Read the model definition and answer for the solid it produces. Units are mm, in the model's axes. Face numbers are marked on the shaded views. A direction names the side the tool comes from. Coordinates: 2 decimals unless noted, no trailing zeros. Write each loop counter-clockwise with the first axis right and the second up, starting at its lowest first coordinate (ties: lowest second). Pieces come first, ordered by that corner, then holes.
(1) The part is cut by section C-C, the plane z = 2.15. Determine the outline of the cut face in (x, y), and give its area (3 significant figures).
(2) The part is cut by section A-A, the plane x = 0.75. Determine the outline of the cut face in (y, z), and give its area (3 significant figures).
(3) Which of the six approach directions +Z, -Z, +X, -X, +Y, -Y give full straight-line access (tool end or side, diameter ignored) to the marked faces 4, 5 and 6?
(4) Straight lines are drawn through the part: line 1 along X through (y, z) = (5.25, 2.4); line 2 along Z through (x, y) = (-6, -1). For each, find the intervals that lie inside material, in ascending order.
(5) Given pin 1 (0.5 mm diameter, centred on x = 1.5, z = 2.5, fed in from +Y); pin 2 (4 mm diameter, centred on x = -1, y = -2, fed in from +Z), each flat-ended and moving along its own axis, determine where each tip first touches the part or whether it passes through.
(6) Determine the mould class of the marked faces 1, 2 and 3 for opening direction X: pulls with the +X half, pulls with the -X half, needs draft (parallel to the pull), parting line crosses it, or undercut.
(7) The part is cut by section B-B, the plane y = -3. Determine the outline of the cut face in (x, z).
Autodesk Fusion 360 part; units mm, degrees
sketch "Sketch1" plane through (0, 0, 0) normal (0, 0, 1) x (1, 0, 0)
  line L0 (-7.9, 7.9) -> (7.9, 7.9)
  line L1 (7.9, 7.9) -> (7.9, -7.9)
  line L2 (7.9, -7.9) -> (-7.9, -7.9)
  line L3 (-7.9, -7.9) -> (-7.9, 7.9)
  line L4 (-7.9, 7.9) -> (7.9, -7.9) construction
  line L5 (7.9, 7.9) -> (-7.9, -7.9) construction
  dimension "d1" = 15.8
extrude "Extrude1" add sketch "Sketch1" along normal blind 3.3
shell "Shell1" thickness 1.55 removed faces 1 at (-2.6333, 2.6333, 3.3)
fillet "Fillet1" radius 2 4 edges at (7.9, 7.9, 1.65) (7.9, -7.9, 1.65) (-7.9, -7.9, 1.65) (-7.9, 7.9, 1.65)
chamfer "Chamfer1" distance 0.4 angle 45 8 edges at (7.9, 0, 0) (7.3142, -7.3142, 0) (0, -7.9, 0) (-7.3142, -7.3142, 0) (-7.9, 0, 0) (-7.3142, 7.3142, 0) (0, 7.9, 0) (7.3142, 7.3142, 0)
chamfer "Chamfer2" distance 0.2 angle 45 4 edges at (-6.35, 0, 3.3) (0, 6.35, 3.3) (6.35, 0, 3.3) (0, -6.35, 3.3)
sketch "Sketch2" plane through (0, 0, 3.3) normal (0, 0, 1) x (1, 0, 0)
  arc A0 (-5.9, 7.9) -> (-7.9, 5.9) centre (-5.9, 5.9) ccw
  line L0 (-7.9, 5.9) -> (-7.9, -5.9)
  arc A1 (-7.9, -5.9) -> (-5.9, -7.9) centre (-5.9, -5.9) ccw
  line L1 (-5.9, -7.9) -> (5.9, -7.9)
  arc A2 (5.9, -7.9) -> (7.9, -5.9) centre (5.9, -5.9) ccw
  line L2 (7.9, -5.9) -> (7.9, 5.9)
  arc A3 (7.9, 5.9) -> (5.9, 7.9) centre (5.9, 5.9) ccw
  line L3 (5.9, 7.9) -> (-5.9, 7.9)
  line L4 (-6.55, -6.55) -> (-6.55, 6.55)
  line L5 (-6.55, 6.55) -> (6.55, 6.55)
  line L6 (6.55, 6.55) -> (6.55, -6.55)
  line L7 (6.55, -6.55) -> (-6.55, -6.55)
  line L8 (0, 0) -> (0, 7.9) construction
  line L9 (2, 6.0755) -> (-2, 6.0755)
  line L10 (-2, 6.0755) -> (-2, 9.7245)
  line L11 (-2, 9.7245) -> (2, 9.7245)
  line L12 (2, 9.7245) -> (2, 6.0755)
  line L13 (2, 6.0755) -> (-2, 9.7245) construction
  line L14 (-2, 6.0755) -> (2, 9.7245) construction
  point P0 (0, 7.9)
  dimension "d9" = 4
extrude "Extrude2" cut sketch "Sketch2" against normal up to surface (1.75 mm away) contours L3 L10 L11 L12 | L3 L5 L10 L12 | L5 L9 L10 L12
fillet "Fillet2" radius 1 2 edges at (-2, 7.125, 1.55) (2, 7.125, 1.55)
chamfer "Chamfer3" distance 0.2 angle 45 2 edges at (2, 7.225, 3.3) (-2, 7.225, 3.3)
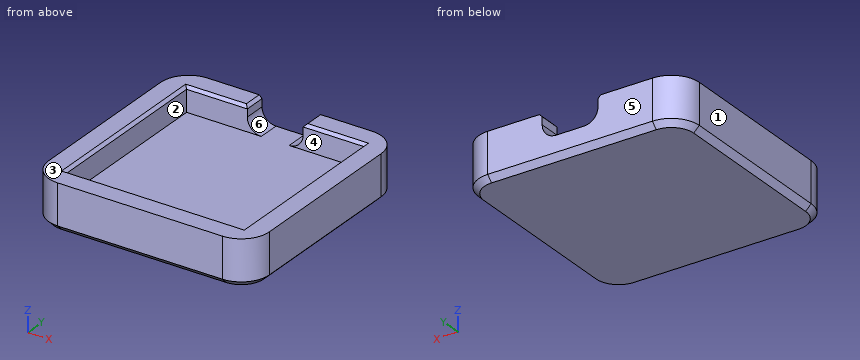
Computed:
1. outline: (-7.9, -5.9) arc R2 ccw to (-5.9, -7.9) - (5.9, -7.9) arc R2 ccw to (7.9, -5.9) - (7.9, 5.9) arc R2 ccw to (5.9, 7.9) - (1.92, 7.9) - (1.92, 6.35) - (6.35, 6.35) - (6.35, -6.35) - (-6.35, -6.35) - (-6.35, 6.35) - (-1.92, 6.35) - (-1.92, 7.9) - (-5.9, 7.9) arc R2 ccw to (-7.9, 5.9) - close
1. area: 79.0 mm2
2. outline: (-7.9, 0.4) - (-7.5, 0) - (7.5, 0) - (7.9, 0.4) - (7.9, 1.55) - (-6.35, 1.55) - (-6.35, 3.1) - (-6.55, 3.3) - (-7.9, 3.3) - close
2. area: 27.0 mm2
3. face 4: +Z
3. face 5: +Z, -Z, +X, -X, +Y
3. face 6: +Z, +Y
4. line 1: x = -7.9 to -6.35, 6.35 to 7.9
4. line 2: z = 0 to 1.55
5. pin 1: stops at y = -6.35
5. pin 2: stops at z = 1.55
6. face 1: pulls with the -X half
6. face 2: undercut
6. face 3: needs draft
7. outline: (-7.9, 0.4) - (-7.5, 0) - (7.5, 0) - (7.9, 0.4) - (7.9, 3.3) - (6.55, 3.3) - (6.35, 3.1) - (6.35, 1.55) - (-6.35, 1.55) - (-6.35, 3.1) - (-6.55, 3.3) - (-7.9, 3.3) - close
